Geometry: final body of the model. Coordinates: model frame, mm. A direction names the side the tool comes from. Give positions to 0.01 mm unless a question says otherwise; leave off trailing zeros. Write each loop counter-clockwise with the first axis right and the second up, starting at its lowest first coordinate (ties: lowest second). Pieces come first, ordered by that corner, then holes. Notation, with made-up numbers: (24.5, -6.5) -> (63.5, -6.5) arc R19 cw to (63.5, 29.5) -> close; hole circle Ø2 at (49.25, 5). An arc over 180 degrees is marked (long way). Answer in a Markdown table with one row per item. Add a question column.
Item 1: Material intervals for probe 1 along X at (y, z) = (12, 0.55); probe 2 along Z at (x, y) = (2.25, 14.5), sorted ascending. Write a range as from..to.
Item 2: Section query A-A on y = 12. Output: boundary loops of the cut face in (x, z), plus the area to 3 significant figures.
Item 3: Section query D-D on x = 1.25. Output: boundary loops of the cut face in (y, z), plus the area to 3 significant figures.
Item 4: Draft query along Y for faces 1 (the flat face through (4, 4, 2)), 2 (the flat face through (4, 4, 7)), 3 (the flat face through (8, 0, 3)). Return one class per face: +Y half, -Y half, draft (parallel to the pull), parting line (faces both ways), or undercut.
Item 5: First-contact query: P1, Ø1.3, axis at x = 12.5, y = 13, coming from the -Z side; P2, Ø1.5, axis at x = 9.5, y = 9.5, coming from the +Z side. Flat tips, straight axial feed; report the tip coordinate or a pass-through.
Item 6: Section query B-B on z = 1.5. Output: boundary loops of the cut face in (x, y).
Item 7: Access query for faces 4 (the flat face through (12, 12, 2)), 5 (the flat face through (0, 8, 3)), 6 (the cylindrical face through (3.74, 13.983, 6.493)). Directions: +Z, -Z, +X, -X, +Y, -Y. A direction counts if a zero-diameter tool reaches every point of the face in a straight line with its end or side. Return the directions, or none.
```python
from build123d import *

# Parameters (mm, degrees)
CYLINDER007_R     = 2.2
CYLINDER007_DEPTH = 7
CYLINDER005_R     = 2.2
CYLINDER005_DEPTH = 7
CYLINDER006_R     = 2.2
CYLINDER006_DEPTH = 7
CYLINDER004_R     = 2.2
CYLINDER004_DEPTH = 7
CYLINDER_R        = 2
CYLINDER_DEPTH    = 7
CYLINDER001_R     = 2
CYLINDER001_DEPTH = 7
CYLINDER002_R     = 2
CYLINDER002_DEPTH = 7
CYLINDER003_R     = 2
CYLINDER003_DEPTH = 7
BOX_W             = 16
BOX_H             = 16
BOX_DEPTH         = 6


with BuildPart() as cylinder007:
    # Cylinder007 → Cylinder007 (new body)
    with BuildSketch(Plane(origin=(12, 12, -5), x_dir=(1, 0, 0), z_dir=(0, 0, 1))):
        Circle(CYLINDER007_R)
    extrude(amount=CYLINDER007_DEPTH)


with BuildPart() as cylinder005:
    # Cylinder005 → Cylinder005 (new body)
    with BuildSketch(Plane(origin=(4, 12, -5), x_dir=(1, 0, 0), z_dir=(0, 0, 1))):
        Circle(CYLINDER005_R)
    extrude(amount=CYLINDER005_DEPTH)


with BuildPart() as cylinder006:
    # Cylinder006 → Cylinder006 (new body)
    with BuildSketch(Plane(origin=(12, 4, -5), x_dir=(1, 0, 0), z_dir=(0, 0, 1))):
        Circle(CYLINDER006_R)
    extrude(amount=CYLINDER006_DEPTH)


with BuildPart() as fusion001:
    # Cylinder004 → Cylinder004 (new body)
    with BuildSketch(Plane(origin=(4, 4, -5), x_dir=(1, 0, 0), z_dir=(0, 0, 1))):
        Circle(CYLINDER004_R)
    extrude(amount=CYLINDER004_DEPTH)

    # Fusion001: union Cylinder007, Cylinder005, Cylinder006
    add(cylinder007.part)
    add(cylinder005.part)
    add(cylinder006.part)


with BuildPart() as cylinder:
    # Cylinder → Cylinder (new body)
    with BuildSketch(Plane(origin=(4, 4, 0), x_dir=(1, 0, 0), z_dir=(0, 0, 1))):
        Circle(CYLINDER_R)
    extrude(amount=CYLINDER_DEPTH)


with BuildPart() as cylinder001:
    # Cylinder001 → Cylinder001 (new body)
    with BuildSketch(Plane(origin=(12, 4, 0), x_dir=(1, 0, 0), z_dir=(0, 0, 1))):
        Circle(CYLINDER001_R)
    extrude(amount=CYLINDER001_DEPTH)


with BuildPart() as cylinder002:
    # Cylinder002 → Cylinder002 (new body)
    with BuildSketch(Plane(origin=(12, 12, 0), x_dir=(1, 0, 0), z_dir=(0, 0, 1))):
        Circle(CYLINDER002_R)
    extrude(amount=CYLINDER002_DEPTH)


with BuildPart() as cylinder003:
    # Cylinder003 → Cylinder003 (new body)
    with BuildSketch(Plane(origin=(4, 12, 0), x_dir=(1, 0, 0), z_dir=(0, 0, 1))):
        Circle(CYLINDER003_R)
    extrude(amount=CYLINDER003_DEPTH)


with BuildPart() as cut:
    # Box → Box (new body)
    with BuildSketch(Plane.XY):
        with Locations((8, 8)):
            Rectangle(BOX_W, BOX_H)
    extrude(amount=BOX_DEPTH)

    # Fusion: union Cylinder, Cylinder001, Cylinder002, Cylinder003
    add(cylinder.part)
    add(cylinder001.part)
    add(cylinder002.part)
    add(cylinder003.part)

    # Cut: cut Fusion001
    add(fusion001.part, mode=Mode.SUBTRACT)


solid = cut.part
```
Findings below:
| question | item | result |
|---|---|---|
| 1 | probe 1 | x = 0..1.8, 6.2..9.8, 14.2..16 |
| 1 | probe 2 | z = 0..6 |
| 2 | outline | (0, 0) -> (1.8, 0) -> (1.8, 2) -> (6.2, 2) -> (6.2, 0) -> (9.8, 0) -> (9.8, 2) -> (14.2, 2) -> (14.2, 0) -> (16, 0) -> (16, 6) -> (14, 6) -> (14, 7) -> (10, 7) -> (10, 6) -> (6, 6) -> (6, 7) -> (2, 7) -> (2, 6) -> (0, 6) -> close |
| 2 | area | 86.4 mm^2 |
| 3 | outline | (0, 0) -> (16, 0) -> (16, 6) -> (0, 6) -> close |
| 3 | area | 96.0 mm^2 |
| 4 | face 1 | undercut |
| 4 | face 2 | draft |
| 4 | face 3 | -Y half |
| 5 | P1 | stops at z = 2 |
| 5 | P2 | stops at z = 6 |
| 6 | outline | (0, 0) -> (16, 0) -> (16, 16) -> (0, 16) -> close; hole circle Ø4.4 at (4, 4); hole circle Ø4.4 at (4, 12); hole circle Ø4.4 at (12, 4); hole circle Ø4.4 at (12, 12) |
| 7 | face 4 | -Z |
| 7 | face 5 | +Z, -Z, -X, +Y, -Y |
| 7 | face 6 | +Z |
